from build123d import *

# Parameters (mm, degrees)
SKETCH1_R           = 2.54
SKETCH1_R_2         = 1.797730585
BOSS_EXTRUDE1_DEPTH = 6.35
CUT_EXTRUDE1_DEPTH  = 92.800885072
FILLET1_R           = 6.35


with BuildPart() as part:
    # Sketch1 → Boss-Extrude1 (new body)
    with BuildSketch(Plane.XY):
        Polygon((25.4, 0), (76.2, 25.4), (76.2, 50.8), (0, 50.8), (0, 0), align=None)
        with Locations((12.7, 12.7)):
            Circle(SKETCH1_R, mode=Mode.SUBTRACT)
        with Locations((69.85, 44.45)):
            Circle(SKETCH1_R_2, mode=Mode.SUBTRACT)
        with Locations((57.15, 44.45)):
            Circle(SKETCH1_R_2, mode=Mode.SUBTRACT)
        with Locations((44.45, 44.45)):
            Circle(SKETCH1_R_2, mode=Mode.SUBTRACT)
        with Locations((31.75, 44.45)):
            Circle(SKETCH1_R_2, mode=Mode.SUBTRACT)
        with Locations((19.05, 44.45)):
            Circle(SKETCH1_R_2, mode=Mode.SUBTRACT)
        with Locations((6.35, 44.45)):
            Circle(SKETCH1_R_2, mode=Mode.SUBTRACT)
        with Locations((57.15, 31.75)):
            Circle(SKETCH1_R_2, mode=Mode.SUBTRACT)
        with Locations((44.45, 31.75)):
            Circle(SKETCH1_R_2, mode=Mode.SUBTRACT)
        with Locations((31.75, 31.75)):
            Circle(SKETCH1_R_2, mode=Mode.SUBTRACT)
        with Locations((19.05, 31.75)):
            Circle(SKETCH1_R_2, mode=Mode.SUBTRACT)
        with Locations((6.35, 31.75)):
            Circle(SKETCH1_R_2, mode=Mode.SUBTRACT)
        with Locations((69.85, 31.75)):
            Circle(SKETCH1_R_2, mode=Mode.SUBTRACT)
    extrude(amount=BOSS_EXTRUDE1_DEPTH)

    # Sketch2 → Cut-Extrude1 (cut, through all)
    with BuildSketch(Plane.XY.offset(6.35)):
        Polygon((21.59, 0), (21.59, 2.54), (27.65106415, 16.522886017), (44.145936938, 9.372968469), (25.4, 0), align=None)
    extrude(amount=-CUT_EXTRUDE1_DEPTH, mode=Mode.SUBTRACT)

    # Fillet1
    # the kernel refuses this fillet: 6.35 mm, written as the material it adds along each edge
    with BuildSketch(Plane(origin=(27.65106415, 16.522886017, 6.35), x_dir=(0.9175122058614823, -0.397707621369263, 0), z_dir=(0, 0, -1))) as fillet1_piece_1:
        with BuildLine():
            CenterArc((FILLET1_R, FILLET1_R), FILLET1_R, 180, 90)
            Line((0, FILLET1_R), (0, 0))
            Line((0, 0), (FILLET1_R, 0))
        make_face()
    extrude(amount=6.35)
    # the kernel refuses this fillet: 6.35 mm, written as the material it takes off along each edge
    with BuildSketch(Plane(origin=(44.145936938, 9.372968469, 13.752634073), x_dir=(0.8944271909999154, 0.4472135954999589, 0), z_dir=(0, 0, -1))) as fillet1_2_piece_1:
        with BuildLine():
            CenterArc((FILLET1_R * 0.466307658155, -FILLET1_R), FILLET1_R, 90, 50)
            Line((-FILLET1_R * 0.299736784964, -FILLET1_R * 0.357212390313), (0, 0))
            Line((0, 0), (FILLET1_R * 0.466307658155, 0))
        make_face()
    extrude(amount=21.155268146, mode=Mode.SUBTRACT)
    with BuildSketch(Plane(origin=(76.2, 25.4, -9.811289571), x_dir=(-0.8944271909999166, -0.4472135954999565, 0), z_dir=(0, 0, 1))) as fillet1_2_piece_2:
        with BuildLine():
            CenterArc((FILLET1_R * 0.61803398875, -FILLET1_R), FILLET1_R, 90, 63.434948823)
            Line((-FILLET1_R * 0.27639320225, -FILLET1_R * 0.5527864045), (0, 0))
            Line((0, 0), (FILLET1_R * 0.61803398875, 0))
        make_face()
    extrude(amount=25.972579143, mode=Mode.SUBTRACT)
    with BuildSketch(Plane(origin=(76.2, 50.8, -15.875), x_dir=(0, -1, 0), z_dir=(0, 0, 1))) as fillet1_2_piece_3:
        with BuildLine():
            CenterArc((FILLET1_R, -FILLET1_R), FILLET1_R, 90, 90)
            Line((0, -FILLET1_R), (0, 0))
            Line((0, 0), (FILLET1_R, 0))
        make_face()
    extrude(amount=38.1, mode=Mode.SUBTRACT)
    with BuildSketch(Plane(origin=(0, 50.8, -15.875), x_dir=(0, -1, 0), z_dir=(0, 0, 1)), Plane(origin=(0, 0, -15.875), x_dir=(1, 0, 0), z_dir=(0, 0, 1))) as fillet1_2_piece_4:
        with BuildLine():
            CenterArc((FILLET1_R, FILLET1_R), FILLET1_R, 180, 90)
            Line((0, FILLET1_R), (0, 0))
            Line((0, 0), (FILLET1_R, 0))
        make_face()
    extrude(amount=38.1, mode=Mode.SUBTRACT)
    with BuildSketch(Plane(origin=(21.59, 0, 19.05), x_dir=(0, 1, 0), z_dir=(0, 0, -1))) as fillet1_2_piece_5:
        with BuildLine():
            CenterArc((6.35, -5.08), FILLET1_R, 126.869897646, 53.130102354)
            Line((0, -5.08), (0, 0))
            Line((0, 0), (2.54, 0))
        make_face()
    extrude(amount=31.75, mode=Mode.SUBTRACT)


solid = part.part
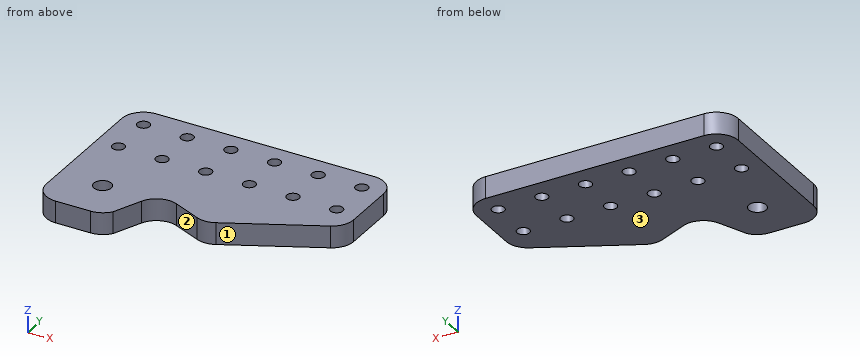
Could you check a few things on this model? Use its own coordinates, in mm. Face numbers are marked on the shaded views. Coordinates: 2 decimals unless noted, no trailing zeros. Write each loop counter-clockwise with the first axis right and the second up, starting at its lowest first coordinate (ties: lowest second). Pieces come first, ordered by that corner, then holes. Notation, with made-up numbers: (41, -1) - (87, -1) arc R21 cw to (87, 32) - close; hole circle Ø4 at (-22.5, 5.25). An arc over 180 degrees is marked (long way). Put each result on its own line as item: value. Start each with the question number.
Q1. I want a section at A-A on y = 31.75. Write out the boundary of the cut face in (x, z), plus the area to 3 significant figures.
Q2. I want a section at C-C on z = 5.25. Count the separate pieces of the cut face and the enclosed holes in it, plus the area to 3 significant figures.
Q3. I want a section at D-D on x = 44.45. Write out the boundary of the cut face in (y, z).
Q4. I'm going to push a flat-ended pin straight in: P1, Ø6, axis at x = 19.05, y = 31.75, coming from the +Z side. Where does the tip first touch, or does it pass through?
Q5. Please list where these lines run through material, in increasing order: L1, parallel to Y at x = 6.35, z = 1.5; L2, parallel to Y at x = 33, z = 3.5; L3, parallel to X at y = 11, z = 2.
Q6. I want a section at B-B on x = 12.7. Write out the boundary of the cut face in (y, z).
Q7. Thinking about a two-plate mould opening in X: for the marked faces 1, 2 and 3, which applies, pulls with the +X half, pulls with the -X half, needs draft (parallel to the pull), parting line crosses it, or undercut?
Checks:
1. outline: (0, 0) - (4.55, 0) - (4.55, 6.35) - (0, 6.35) - close; (8.15, 0) - (17.25, 0) - (17.25, 6.35) - (8.15, 6.35) - close; (20.85, 0) - (29.95, 0) - (29.95, 6.35) - (20.85, 6.35) - close; (33.55, 0) - (42.65, 0) - (42.65, 6.35) - (33.55, 6.35) - close; (46.25, 0) - (55.35, 0) - (55.35, 6.35) - (46.25, 6.35) - close; (58.95, 0) - (68.05, 0) - (68.05, 6.35) - (58.95, 6.35) - close; (71.65, 0) - (76.2, 0) - (76.2, 6.35) - (71.65, 6.35) - close
1. area: 347 mm²
2. separate pieces: 1
2. enclosed holes: 13
2. area: 2,880 mm²
3. outline: (10.05, 0) - (29.95, 0) - (29.95, 6.35) - (10.05, 6.35) - close; (33.55, 0) - (42.65, 0) - (42.65, 6.35) - (33.55, 6.35) - close; (46.25, 0) - (50.8, 0) - (50.8, 6.35) - (46.25, 6.35) - close
4. P1: z = 6.35
5. L1: 0 to 29.95, 33.55 to 42.65, 46.25 to 50.8
5. L2: 14.18 to 30.46, 33.04 to 43.16, 45.74 to 50.8
5. L3: 0 to 10.81, 14.59 to 25.27, 40.39 to 47.4
6. outline: (0, 0) - (10.16, 0) - (10.16, 6.35) - (0, 6.35) - close; (15.24, 0) - (50.8, 0) - (50.8, 6.35) - (15.24, 6.35) - close
7. face 1: pulls with the +X half
7. face 2: undercut
7. face 3: needs draft
